For this review, take the finished solid that the model builds, in its own axes (mm). A direction names the side the tool comes from. Round coordinates to 2 decimals unless told otherwise and drop trailing zeros. Loops run counter-clockwise (first coordinate to the right, second up) from the corner with the lowest first, then second, coordinate; pieces in that order, holes last. Notation, with made-up numbers: M 27.25,85 L 75.25,85 A10 ccw 75.25,99 Z; hole C -32,-31 d5. An arc over 180 degrees is marked long. One line per question, with ' | ' between items. Start each with the question number.
1) We need section B-B (y = 30). Give the boundary of the cut face in (x, z).
2) For probe 1 along Z at (x, y) = (8, 44); probe 2 along Z at (x, y) = (-14, 56.5); probe 3 along Y at (x, z) = (-10, -4.5), list the stretches that pass through material, from the lowest coordinate up. Write a range as from..to.
3) We need section D-D (z = 0). Give the boundary of the cut face in (x, y).
4) We need section C-C (x = 2.5). State how many separate pieces and enclosed holes the cut face has, and give its area (3 significant figures).
5) For pin 1 Ø1.1 at (x, z) = (-16, 17) entering from -Y; pin 2 Ø8 at (y, z) = (31, 19.5) entering from +X; pin 3 Ø3 at (x, z) = (-3, 14) entering from +Y; pin 4 Ø12 at (x, z) = (4.5, -8.5) entering from +Y, all flat-tipped, find the tip position at first contact; note any pin that passes through.
6) For faces 4 (the face through (8, 0, -13)), 5 (the face through (-1, 58, 16.607)), list the 3-axis set-ups (+Z, -Z, +X, -X, +Y, -Y) from which the entire face can be reached by the end or side of a thin tool; tool diameter is ignored.
7) Mouldability with a two-part tool opening along X and no side actions: class faces 1 (the face through (7.25, 41.11, 20.14)), 2 (the face through (14.899, 27, 20)), 3 (the face through (-0.877, 6.426, 16.104)) as pulls with the +X half, pulls with the -X half, needs draft (parallel to the pull), parting line crosses it, or undercut.
8) We need section A-A (y = 39). Give the boundary of the cut face in (x, z).
```python
from build123d import *

# Parameters (mm, degrees)
SKETCH1_W           = 32
SKETCH1_H           = 71.5
BOSS_EXTRUDE1_DEPTH = 5
SKETCH2_W           = 32
SKETCH2_H           = 5
BOSS_EXTRUDE2_DEPTH = 45
BOSS_EXTRUDE3_DEPTH = 6
SKETCH4_R           = 5
SKETCH4_R_2         = 1.25
CUT_EXTRUDE1_DEPTH  = 99.796262783
SKETCH5_R           = 5
SKETCH5_R_2         = 1.25
CUT_EXTRUDE2_DEPTH  = 84.89844385
FILLET1_R           = 5
BOSS_EXTRUDE4_DEPTH = 5
FILLET2_R           = 1


with BuildPart() as part:
    # Sketch1 → Boss-Extrude1 (new body)
    with BuildSketch(Plane(origin=(0, 0, 0), x_dir=(1, 0, 0), z_dir=(0, 1, 0))):
        with Locations((-1.101214575, 13.142712551)):
            Rectangle(SKETCH1_W, SKETCH1_H)
    extrude(amount=BOSS_EXTRUDE1_DEPTH)

    # Sketch2 → Boss-Extrude2 (add)
    with BuildSketch(Plane(origin=(0, 5, 0), x_dir=(1, 0, 0), z_dir=(0, 1, 0))):
        with Locations((-1.101214575, -20.107287449)):
            Rectangle(SKETCH2_W, SKETCH2_H)
    boss_extrude2 = extrude(amount=BOSS_EXTRUDE2_DEPTH)

    # Mirror1: Boss-Extrude2 across plane
    add(boss_extrude2.mirror(Plane(origin=(0, 0, -13.142712551), x_dir=(1, 0, 0), z_dir=(0, 0, -1))))

    # Sketch3 → Boss-Extrude3 (add)
    with BuildSketch(Plane.XY.offset(22.607287449)):
        with BuildLine():
            Line((-17.101214575, 50), (14.898785425, 50))
            ThreePointArc((14.898785425, 50), (-1.101214575, 66), (-17.101214575, 50))
        make_face()
    boss_extrude3 = extrude(amount=-BOSS_EXTRUDE3_DEPTH)

    # Mirror3: Boss-Extrude3 across plane
    add(boss_extrude3.mirror(Plane(origin=(0, 0, -13.142712551), x_dir=(1, 0, 0), z_dir=(0, 0, -1))))

    # Sketch4 → Cut-Extrude1 (cut, through all)
    with BuildSketch(Plane.XY.offset(22.607287449)):
        with Locations((-1.101214575, 50)):
            Circle(SKETCH4_R)
        with Locations((-1.101214575, 61)):
            Circle(SKETCH4_R_2)
        with Locations((6.676960018, 57.778174593)):
            Circle(SKETCH4_R_2)
        with Locations((9.898785425, 50)):
            Circle(SKETCH4_R_2)
        with Locations((6.676960018, 42.221825407)):
            Circle(SKETCH4_R_2)
        with Locations((-1.101214575, 39)):
            Circle(SKETCH4_R_2)
        with Locations((-8.879389168, 42.221825407)):
            Circle(SKETCH4_R_2)
        with Locations((-12.101214575, 50)):
            Circle(SKETCH4_R_2)
        with Locations((-8.879389168, 57.778174593)):
            Circle(SKETCH4_R_2)
    extrude(amount=-CUT_EXTRUDE1_DEPTH, mode=Mode.SUBTRACT)

    # Sketch5 → Cut-Extrude2 (cut, through all)
    with BuildSketch(Plane(origin=(0, 0, 0), x_dir=(-1, 0, 0), z_dir=(0, -1, 0))):
        with Locations(Location((1.101214575, 13.142712551, 0), (0, 0, 90))):
            Circle(SKETCH5_R)
        with Locations(Location((1.101214575, 24.142712551, 0), (0, 0, 90))):
            Circle(SKETCH5_R_2)
        with Locations(Location((8.879389168, 20.920887144, 0), (0, 0, 90))):
            Circle(SKETCH5_R_2)
        with Locations(Location((12.101214575, 13.142712551, 0), (0, 0, 90))):
            Circle(SKETCH5_R_2)
        with Locations(Location((8.879389168, 5.364537958, 0), (0, 0, 90))):
            Circle(SKETCH5_R_2)
        with Locations(Location((1.101214575, 2.142712551, 0), (0, 0, 90))):
            Circle(SKETCH5_R_2)
        with Locations(Location((-6.676960018, 5.364537958, 0), (0, 0, 90))):
            Circle(SKETCH5_R_2)
        with Locations(Location((-9.898785425, 13.142712551, 0), (0, 0, 90))):
            Circle(SKETCH5_R_2)
        with Locations(Location((-6.676960018, 20.920887144, 0), (0, 0, 90))):
            Circle(SKETCH5_R_2)
    extrude(amount=-CUT_EXTRUDE2_DEPTH, mode=Mode.SUBTRACT)

    # Fillet1
    fillet1_edges = [part.edges().sort_by_distance(p)[0] for p in [
        (-1.101214575, 5, 17.607287449),
        (-1.101214575, 5, -43.892712551),
    ]]
    fillet(fillet1_edges, radius=FILLET1_R)

    # Sketch6 → Boss-Extrude4 (add)
    with BuildSketch(Plane.XZ):
        with BuildLine():
            Line((14.898785425, 22.607287449), (14.898785425, -48.892712551))
            ThreePointArc((14.898785425, -48.892712551), (34.663505701, -13.142712551), (14.898785425, 22.607287449))
        make_face()
    extrude(amount=-BOSS_EXTRUDE4_DEPTH)

    # Fillet2
    fillet2_edges = [part.edges().sort_by_distance(p)[0] for p in [
        (-1.101214575, 66, -42.892712551),
    ]]
    fillet(fillet2_edges, radius=FILLET2_R)


solid = part.part
```
Answers below:
1) outline: M -17.1,-48.89 L 14.9,-48.89 L 14.9,-43.89 L -17.1,-43.89 Z; M -17.1,17.61 L 14.9,17.61 L 14.9,22.61 L -17.1,22.61 Z
2) probe 1: -48.89..-43.89, 17.61..22.61 | probe 2: -48.89..-42.89, 16.61..22.61 | probe 3: 0..5
3) outline: M -17.1,0 L 32.57,0 L 32.57,5 L -17.1,5 Z
4) separate pieces: 4 | enclosed holes: 0 | area: 894 mm^2
5) pin 1: y = 0 | pin 2: x = 14.9 | pin 3: y = 5.92 | pin 4: y = 5
6) face 4: +Z, -Z, +X, -X, -Y | face 5: +X, -X, +Y
7) face 1: undercut | face 2: pulls with the +X half | face 3: needs draft
8) outline: M -17.1,-48.89 L -2.35,-48.89 L -2.35,-43.89 L -17.1,-43.89 Z; M -17.1,17.61 L -2.35,17.61 L -2.35,22.61 L -17.1,22.61 Z; M 0.15,-48.89 L 14.9,-48.89 L 14.9,-43.89 L 0.15,-43.89 Z; M 0.15,17.61 L 14.9,17.61 L 14.9,22.61 L 0.15,22.61 Z
